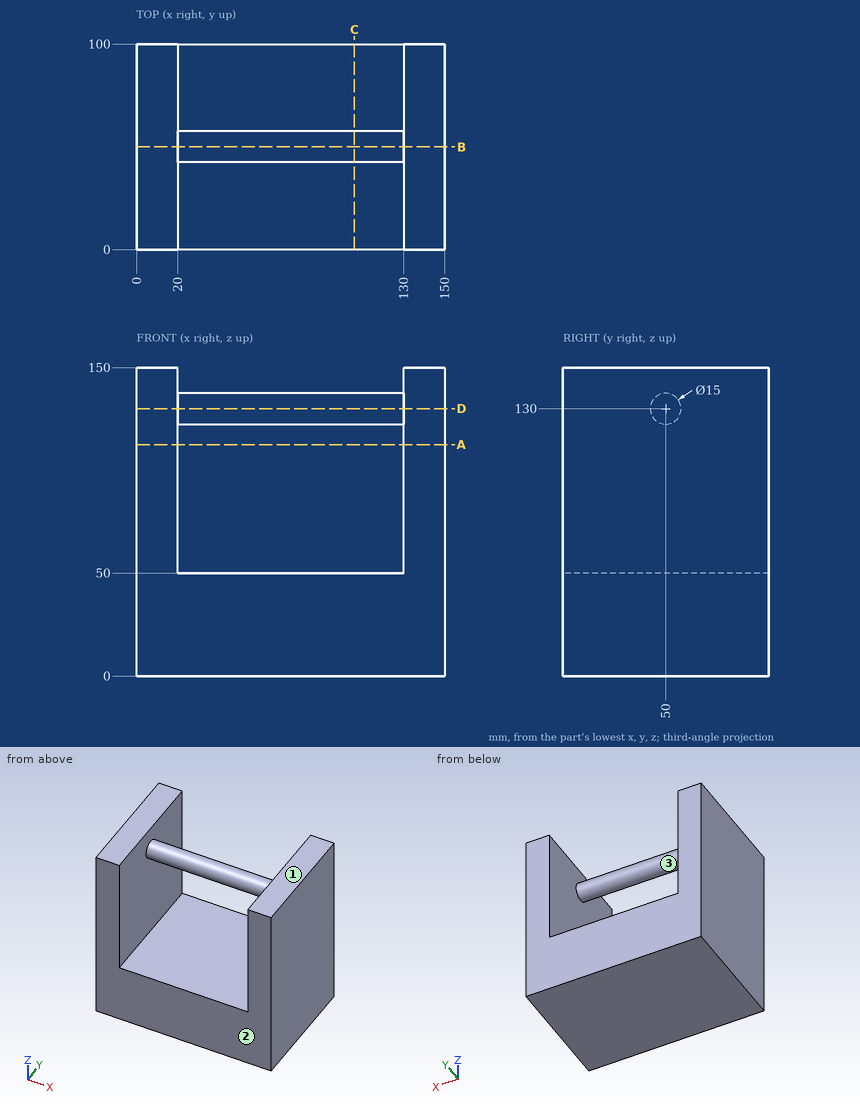
Answer from the drawing. Dimensions are ordinates in mm from the lowest x, y and z of the part. Round coordinates to 2 decimals unless told otherwise and drop trailing zeros. Write each loop counter-clockwise with the first axis right and the second up, starting at its lowest first coordinate (ties: lowest second). Pieces come first, ordered by that corner, then holes. Notation, with made-up numbers: (-26, 56.25) -> (-4, 56.25) arc R25 cw to (-4, 89.25) -> close; hole circle Ø9 at (8, 38.5). An arc over 180 degrees is marked (long way). Answer in a Markdown table with one row per item. Add a question column.
1) Consider line 1 (X direction, y = 91, z = 138); line 2 (Z direction, x = 56, y = 29); line 3 (Z direction, x = 99, y = 56). Determine where each line is inside the solid, lowest interval first.
2) Find section A-A, the plane z = 112.5. Determine the outline of the cut face in (x, y), and give its area (3 significant figures).
3) Given P1, Ø10, axis at y = 51, z = 75, coming from the -X side; P2, Ø2, axis at x = 101, y = 12, coming from the +Z side, each flat-ended and moving along its own axis, determine where each tip first touches the part or whether it passes through.
4) Find section D-D, the plane z = 130. Determine the outline of the cut face in (x, y).
5) Determine the mould class of the marked faces 1, 2 and 3 for opening direction Z: pulls with the +Z half, pulls with the -Z half, needs draft (parallel to the pull), parting line crosses it, or undercut.
6) Find section C-C, the plane x = 106. Determine the outline of the cut face in (y, z).
7) Find section B-B, the plane y = 50. Determine the outline of the cut face in (x, z).
Findings below:
| question | item | result |
|---|---|---|
| 1 | line 1 | 0 to 20, 130 to 150 |
| 1 | line 2 | 0 to 50 |
| 1 | line 3 | 0 to 50, 125.5 to 134.5 |
| 2 | outline | (0, 0) -> (20, 0) -> (20, 100) -> (0, 100) -> close; (130, 0) -> (150, 0) -> (150, 100) -> (130, 100) -> close |
| 2 | area | 4,000 mm² |
| 3 | P1 | x = 0 |
| 3 | P2 | z = 50 |
| 4 | outline | (0, 0) -> (20, 0) -> (20, 42.5) -> (130, 42.5) -> (130, 0) -> (150, 0) -> (150, 100) -> (130, 100) -> (130, 57.5) -> (20, 57.5) -> (20, 100) -> (0, 100) -> close |
| 5 | face 1 | pulls with the +Z half |
| 5 | face 2 | needs draft |
| 5 | face 3 | undercut |
| 6 | outline | (0, 0) -> (100, 0) -> (100, 50) -> (0, 50) -> close; circle Ø15 at (50, 130) |
| 7 | outline | (0, 0) -> (150, 0) -> (150, 150) -> (130, 150) -> (130, 137.5) -> (20, 137.5) -> (20, 150) -> (0, 150) -> close; hole (20, 50) -> (130, 50) -> (130, 122.5) -> (20, 122.5) -> close |
